Autodesk Inventor part; units mm, degrees
ref_plane "YZ Plane" through (0, 0, 0) normal (1, 0, 0) x (0, 1, 0)
ref_plane "XZ Plane" through (0, 0, 0) normal (0, 1, 0) x (-1, 0, 0)
ref_plane "XY Plane" through (0, 0, 0) normal (0, 0, 1) x (1, 0, 0)
sketch "Sketch1" plane through (0, 0, 0) normal (0, 0, 1) x (1, 0, 0)
  arc A0 (-25.4018, -15) -> (25.4018, -15) centre (0, 0) ccw
  line L0 (2.5, -32) -> (2.5, -39)
  line L1 (2.5, -39) -> (-2.5, -39)
  line L2 (-2.5, -39) -> (-2.5, -32)
  line L3 (-2.5, -32) -> (-2.5, -31.9022)
  line L4 (2.5, -32) -> (2.5, -31.9022)
  arc A1 (-28.2666, -15) -> (-2.5, -31.9022) centre (0, 0) ccw
  arc A2 (2.5, -31.9022) -> (28.2666, -15) centre (0, 0) ccw
  arc A3 (-27.7534, -10) -> (27.7534, -10) centre (0, 0) ccw
  arc A4 (-30.3974, -10) -> (-2.5, -31.9022) centre (0, 0) ccw
  arc A5 (2.5, -31.9022) -> (30.3974, -10) centre (0, 0) ccw
  arc A6 (-29.5, 0) -> (29.5, 0) centre (0, 0) ccw
  line L5 (-32, 0) -> (-29.5, 0)
  line L6 (29.5, 0) -> (32, 0)
  arc A7 (2.5, -31.9022) -> (32, 0) centre (0, 0) ccw
  arc A8 (-32, 0) -> (-2.5, -31.9022) centre (0, 0) ccw
  point P0 (25.4018, -15)
  point P1 (-28.2666, -15)
  point P2 (27.7534, -10)
  point P3 (-30.3974, -10)
  dimension "d43" = 5
  dimension "d64" = 7
extrude "Extrusion8" add sketch "Sketch1" along normal blind 5
properties part number "Clip_TestFitV1"
The model under review builds one solid part; all positions refer to its coordinate system, in mm. A direction names the side the tool comes from. Give positions to 0.01 mm unless a question says otherwise; leave off trailing zeros. Write each loop counter-clockwise with the first axis right and the second up, starting at its lowest first coordinate (ties: lowest second). Pieces come first, ordered by that corner, then holes. Notation, with made-up numbers: M 73.25,76 L 82.25,76 A17 cw 82.25,109 Z; hole C 27,7.5 d4. An arc over 180 degrees is marked long. One line per question, with ' | ' between items. Start each with the question number.
Item 1: Wall thickness on line 1 (X direction, y = -15, z = 1.35); line 2 (X direction, y = -23, z = 3.1); line 3 (Y direction, x = 15, z = 2.3): over which ranges is each line inside the solid? List them lowest first. Write a range as from..to.
Item 2: Draft analysis for pull direction X (two halves, no side actions). For faces 4 (the cylindrical face through (29.07, -5.01, 2.46)), 5 (the cylindrical face through (29.453, -12.51, 2.465)), 6 (the cylindrical face through (-29.423, -12.58, 2.465)), state which applies: released by +X, released by -X, zero draft, split by the parting line, or undercut.
Item 3: For faces 1 (the flat face through (-2.5, -36, 2)), 2 (the cylindrical face through (-29.048, -5.146, 2.465)), 3 (the flat face through (2.5, -36, 2)), list the 3-axis set-ups (+Z, -Z, +X, -X, +Y, -Y) from which the entire face can be reached by the end or side of a thin tool; tool diameter is ignored.
Item 4: For pin 1 (12 mm diameter, centred on x = 22.5, y = -16, fed in from +Z); pin 2 (1.5 mm diameter, centred on y = -37, z = 3, fed in from -X); pin 3 (1.5 mm diameter, centred on y = -13.5, z = 3, fed in from -X); pin 4 (1.5 mm diameter, centred on x = 20.5, z = 3.5, fed in from -Y), all flat-tipped, find the tip position at first contact; note any pin that passes through.
Item 5: We need section B-B on y = -11. Write out the cut boundary in (x, z), plus the area to 3 significant figures.
Item 6: We need section A-A on z = 1.35. Write out the cut boundary in (x, y).
Item 7: We need section D-D on x = -19.5. Write out the cut boundary in (y, z).
Item 8: We need section C-C on y = -4. Write out the cut boundary in (x, z).
Results found:
1) line 1: x = -28.27..-25.4, 25.4..28.27 | line 2: x = -22.25..-18.47, 18.47..22.25 | line 3: y = -28.27..-25.4
2) face 4: undercut | face 5: released by +X | face 6: released by -X
3) face 1: +Z, -Z, -X, -Y | face 2: +Z, -Z, +Y | face 3: +Z, -Z, +X, -Y
4) pin 1: stops at z = 5 | pin 2: stops at x = -2.5 | pin 3: stops at x = -29.35 | pin 4: stops at y = -25.18
5) outline: M -30.05,0 L -27.37,0 L -27.37,5 L -30.05,5 Z; M 27.37,0 L 30.05,0 L 30.05,5 L 27.37,5 Z | area: 26.8 mm2
6) outline: M -32,0 A32 ccw -30.4,-10 A32 ccw -28.27,-15 A32 ccw -2.5,-31.9 L -2.5,-39 L 2.5,-39 L 2.5,-31.9 A32 ccw 28.27,-15 A32 ccw 30.4,-10 A32 ccw 32,0 L 29.5,0 A29.5 cw -25.4,-15 A29.5 cw -27.75,-10 A29.5 cw -29.5,0 Z
7) outline: M -25.37,0 L -22.14,0 L -22.14,5 L -25.37,5 Z
8) outline: M -31.75,0 L -29.23,0 L -29.23,5 L -31.75,5 Z; M 29.23,0 L 31.75,0 L 31.75,5 L 29.23,5 Z
